Geometry: final body of the model. Coordinates: model frame, mm. Face numbers are marked on the shaded views. Give positions to 0.01 mm unless a question says otherwise; leave off trailing zeros. Loops run counter-clockwise (first coordinate to the right, second up) from the corner with the lowest first, then second, coordinate; pieces in that order, holes last. Notation, with made-up numbers: M -23.75,67 L -1.75,67 A19 cw -1.75,84 Z; hole C 5.25,29.25 d10. An arc over 180 degrees is marked long. Put each result on its own line as item: value.
```python
from build123d import *

# Parameters (mm, degrees)
SKETCH2_W             = 80
SKETCH2_H             = 30
SKETCH2_R             = 1.5
SKETCH2_R_2           = 3.4
BOSS_EXTRUDE1_DEPTH   = 2
SKETCH3_W             = 6
SKETCH3_H             = 1.5
BOSS_EXTRUDE2_DEPTH   = 9
SKETCH9_R             = 4
SKETCH9_R_2           = 1.5
BOSS_EXTRUDE4_DEPTH   = 7
SKETCH4_R             = 6
SKETCH4_R_2           = 3.4
BOSS_EXTRUDE3_DEPTH   = 4
SKETCH10_R            = 4
SKETCH10_R_2          = 1.5
CUT_EXTRUDE7_DEPTH    = 7
SKETCH11_W            = 6
SKETCH11_H            = 1.5
CUT_EXTRUDE8_DEPTH    = 11
SKETCH12_W            = 3.3
SKETCH12_H            = 9
BOSS_EXTRUDE5_DEPTH   = 9
CUT_EXTRUDE11_DEPTH   = 1.5
CUT_EXTRUDE12_DEPTH   = 1.5
SKETCH18_R            = 1.55
CUT_EXTRUDE13_DEPTH   = 81
CHAMFER1_SIZE         = 2
CHAMFER1_SIZE2        = 3.464101615
CHAMFER1_PART_2_SIZE  = 2
CHAMFER1_PART_2_SIZE2 = 3.464101615
CHAMFER1_PART_3_SIZE  = 2
CHAMFER1_PART_3_SIZE2 = 3.464101615
CHAMFER1_PART_4_SIZE  = 2
CHAMFER1_PART_4_SIZE2 = 3.464101615


with BuildPart() as part:
    # Sketch2 → Boss-Extrude1 (new body)
    with BuildSketch(Plane(origin=(0, 0, 0), x_dir=(1, 0, 0), z_dir=(0, 1, 0))):
        with Locations((25, 1)):
            Rectangle(SKETCH2_W, SKETCH2_H)
        with Locations(Location((0, 0, 0), (0, 0, 270))):  # turned: the seam where the file's is
            Circle(SKETCH2_R, mode=Mode.SUBTRACT)
        with Locations(Location((50, 0, 0), (0, 0, 270))):  # turned: the seam where the file's is
            Circle(SKETCH2_R, mode=Mode.SUBTRACT)
        with Locations(Location((25, 6, 0), (0, 0, 270))):  # turned: the seam where the file's is
            Circle(SKETCH2_R_2, mode=Mode.SUBTRACT)
    extrude(amount=BOSS_EXTRUDE1_DEPTH)

    # Sketch3 → Boss-Extrude2 (add)
    with BuildSketch(Plane(origin=(0, 2, 0), x_dir=(1, 0, 0), z_dir=(0, 1, 0))):
        Polygon((6, -14), (44, -14), (41, -12.5), (9, -12.5), align=None)
        with Locations((16.5, 15.25)):
            Rectangle(SKETCH3_W, SKETCH3_H)
        with Locations((33.5, 15.25)):
            Rectangle(SKETCH3_W, SKETCH3_H)
    extrude(amount=BOSS_EXTRUDE2_DEPTH)

    # Sketch9 → Boss-Extrude4 (add)
    with BuildSketch(Plane(origin=(0, 2, 0), x_dir=(1, 0, 0), z_dir=(0, 1, 0))):
        with Locations(Location((50, 0, 0), (0, 0, 90))):  # turned: the seam where the file's is
            Circle(SKETCH9_R)
        with Locations(Location((50, 0, 0), (0, 0, 270))):  # turned: the seam where the file's is
            Circle(SKETCH9_R_2, mode=Mode.SUBTRACT)
        with Locations(Location((0, 0, 0), (0, 0, 90))):  # turned: the seam where the file's is
            Circle(SKETCH9_R)
        with Locations(Location((0, 0, 0), (0, 0, 270))):  # turned: the seam where the file's is
            Circle(SKETCH9_R_2, mode=Mode.SUBTRACT)
    extrude(amount=BOSS_EXTRUDE4_DEPTH)

    # Sketch4 → Boss-Extrude3 (add)
    with BuildSketch(Plane.XZ):
        with Locations(Location((25, -6, 0), (0, 0, 270))):  # turned: the seam where the file's is
            Circle(SKETCH4_R)
        with Locations(Location((25, -6, 0), (0, 0, 270))):  # turned: the seam where the file's is
            Circle(SKETCH4_R_2, mode=Mode.SUBTRACT)
    extrude(amount=BOSS_EXTRUDE3_DEPTH)

    # Sketch10 → Cut-Extrude7 (cut)
    with BuildSketch(Plane(origin=(0, 9, 0), x_dir=(1, 0, 0), z_dir=(0, 1, 0))):
        with Locations((50, 0)):
            Circle(SKETCH10_R)
        with Locations(Location((50, 0, 0), (0, 0, 90))):  # turned: the seam where the file's is
            Circle(SKETCH10_R_2, mode=Mode.SUBTRACT)
        Circle(SKETCH10_R)
        with Locations(Location((0, 0, 0), (0, 0, 90))):  # turned: the seam where the file's is
            Circle(SKETCH10_R_2, mode=Mode.SUBTRACT)
    extrude(amount=-CUT_EXTRUDE7_DEPTH, mode=Mode.SUBTRACT)

    # Sketch11 → Cut-Extrude8 (cut)
    with BuildSketch(Plane(origin=(0, 11, 0), x_dir=(1, 0, 0), z_dir=(0, 1, 0))):
        with Locations((33.5, 15.25)):
            Rectangle(SKETCH11_W, SKETCH11_H)
        Polygon((9, -12.5), (6, -14), (44, -14), (41, -12.5), align=None)
        with Locations((16.5, 15.25)):
            Rectangle(SKETCH11_W, SKETCH11_H)
    extrude(amount=-CUT_EXTRUDE8_DEPTH, mode=Mode.SUBTRACT)

    # Sketch12 → Boss-Extrude5 (add)
    with BuildSketch(Plane.XZ):
        with Locations((-13.35, 2.307056314)):
            Rectangle(SKETCH12_W, SKETCH12_H)
        with Locations((63.35, 2.307056314)):
            Rectangle(SKETCH12_W, SKETCH12_H)
    extrude(amount=BOSS_EXTRUDE5_DEPTH)

    # Sketch15 → Cut-Extrude11 (cut)
    with BuildSketch(Plane(origin=(-11.7, 0, 0), x_dir=(0, 0, -1), z_dir=(1, 0, 0))):
        Polygon((-2.307056314, -1.266838493), (-5.107056314, -2.883419246), (-5.107056314, -6.116580754), (-2.307056314, -7.733161507), (0.492943686, -6.116580754), (0.492943686, -2.883419246), align=None)
    extrude(amount=-CUT_EXTRUDE11_DEPTH, mode=Mode.SUBTRACT)

    # Sketch16 → Cut-Extrude12 (cut)
    with BuildSketch(Plane.ZY.offset(-61.7)):
        Polygon((2.307056314, -1.266838493), (-0.492943686, -2.883419246), (-0.492943686, -6.116580754), (2.307056314, -7.733161507), (5.107056314, -6.116580754), (5.107056314, -2.883419246), align=None)
    extrude(amount=-CUT_EXTRUDE12_DEPTH, mode=Mode.SUBTRACT)

    # Sketch18 → Cut-Extrude13 (cut, through all)
    with BuildSketch(Plane.ZY.offset(15)):
        with Locations((2.307056314, -4.5)):
            Circle(SKETCH18_R)
    extrude(amount=-CUT_EXTRUDE13_DEPTH, mode=Mode.SUBTRACT)

    # Chamfer1
    chamfer1_edges = [part.edges().sort_by_distance(p)[0] for p in [
        (-13.35, -9, -2.192943686),
    ]]
    chamfer1_side = [part.faces().sort_by_distance(p)[0] for p in [
        (-13.35, -4.5, -2.192943686),
    ]]
    chamfer(chamfer1_edges, length=CHAMFER1_SIZE, length2=CHAMFER1_SIZE2, reference=chamfer1_side[0])

    # Chamfer1 part 2
    chamfer1_part_2_edges = [part.edges().sort_by_distance(p)[0] for p in [
        (-13.35, -9, 6.807056314),
    ]]
    chamfer1_part_2_side = [part.faces().sort_by_distance(p)[0] for p in [
        (-13.35, -4.5, 6.807056314),
    ]]
    chamfer(chamfer1_part_2_edges, length=CHAMFER1_PART_2_SIZE, length2=CHAMFER1_PART_2_SIZE2, reference=chamfer1_part_2_side[0])

    # Chamfer1 part 3
    chamfer1_part_3_edges = [part.edges().sort_by_distance(p)[0] for p in [
        (63.35, -9, 6.807056314),
    ]]
    chamfer1_part_3_side = [part.faces().sort_by_distance(p)[0] for p in [
        (63.35, -4.5, 6.807056314),
    ]]
    chamfer(chamfer1_part_3_edges, length=CHAMFER1_PART_3_SIZE, length2=CHAMFER1_PART_3_SIZE2, reference=chamfer1_part_3_side[0])

    # Chamfer1 part 4
    chamfer1_part_4_edges = [part.edges().sort_by_distance(p)[0] for p in [
        (63.35, -9, -2.192943686),
    ]]
    chamfer1_part_4_side = [part.faces().sort_by_distance(p)[0] for p in [
        (63.35, -4.5, -2.192943686),
    ]]
    chamfer(chamfer1_part_4_edges, length=CHAMFER1_PART_4_SIZE, length2=CHAMFER1_PART_4_SIZE2, reference=chamfer1_part_4_side[0])


solid = part.part
```
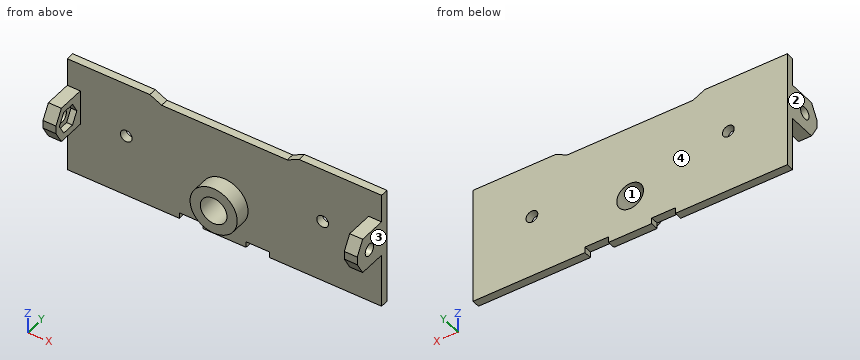
Item 1: Mould query, pull axis X, two halves, no side actions, for the marked faces 1, 2, 3 and 4. Classes: pulls with the +X half, pulls with the -X half, needs draft (parallel to the pull), parting line crosses it, or undercut.
Output values:
face 1: undercut
face 2: pulls with the -X half
face 3: pulls with the +X half
face 4: needs draft
Item 2: Section D-D on x = -10. Output: boundary loops of the cut face in (y, z).
Output values:
outline: M 0,-16 L 2,-16 L 2,14 L 0,14 Z
Item 3: Pin query (flat end, axial travel): pin 1 Ø1.6 at (x, y) = (18, 1.5) entering from -Z; pin 2 Ø1 at (x, y) = (-14, -4) entering from +Z; pin 3 Ø0.6 at (x, y) = (20, 1) entering from +Z. Return the tip coordinate at first contact, or that it passes through.
Output values:
pin 1: z = -14.5
pin 2: z = 6.81
pin 3: z = 12.5
Item 4: Section B-B on z = -6. Output: boundary loops of the cut face in (x, y), then the cut area to 3 significant figures.
Output values:
outline: M -15,0 L 19,0 L 19,-4 L 21.6,-4 L 21.6,2 L -15,2 Z; M 28.4,-4 L 31,-4 L 31,0 L 65,0 L 65,2 L 28.4,2 Z
area: 167 mm²
Item 5: Line query: probe 1 along X at (y, z) = (-2.75, 4); probe 2 along X at (y, z) = (0.5, -5.75); probe 3 along Y at (x, z) = (60, -3). Output: solid intervals per line, ascending. Write a range as [from, to].
Output values:
probe 1: [-15, -13.2], [63.2, 65]
probe 2: [-15, 21.61], [28.39, 65]
probe 3: [0, 2]
Item 6: Section C-C on x = 25. Output: boundary loops of the cut face in (y, z), then the cut area to 3 significant figures.
Output values:
outline: M -4,-12 L 0,-12 L 0,-16 L 2,-16 L 2,-9.4 L -4,-9.4 Z; M -4,-2.6 L 2,-2.6 L 2,12.5 L 0,12.5 L 0,0 L -4,0 Z
area: 64.2 mm²
Item 7: Section A-A on x = 0. Output: boundary loops of the cut face in (y, z).
Output values:
outline: M 0,-16 L 2,-16 L 2,-1.5 L 0,-1.5 Z; M 0,1.5 L 2,1.5 L 2,14 L 0,14 Z
